from build123d import *

# Parameters (mm, degrees)
F1_DEPTH = 41.275
F2_R     = 5.08
F3_R     = 9.525
F4_R     = 6.35
F5_DEPTH = 55.5635
F6_R     = 6.35
F7_DEPTH = 25.4
F8_W     = 203.2
F8_H     = 76.2
F8_R     = 7.9375
F9_DEPTH = 6.35


with BuildPart() as f1:
    # F0 (on Front) → F1 (new body, symmetric)
    with BuildSketch(Plane.XZ):
        Polygon((21.43125, 21.43125), (21.43125, -21.43125), (-21.43125, -21.43125), (-21.43125, 21.43125), (-27.78125, 21.43125), (-27.78125, -21.43125), (-27.78125, -27.78125), (-21.43125, -27.78125), (21.43125, -27.78125), (27.78125, -27.78125), (27.78125, -21.43125), (27.78125, 21.43125), align=None)
    extrude(amount=F1_DEPTH, both=True)

    # F2
    f2_edges = [f1.edges().sort_by_distance(p)[0] for p in [
        (-21.43125, 0, -21.43125),
        (21.43125, 0, -21.43125),
    ]]
    fillet(f2_edges, radius=F2_R)

    # F3
    f3_edges = [f1.edges().sort_by_distance(p)[0] for p in [
        (-27.78125, 0, -27.78125),
        (27.78125, 0, -27.78125),
    ]]
    fillet(f3_edges, radius=F3_R)

    # F4 (on face) → F5 (cut, through all)
    with BuildSketch(Plane.YZ.offset(27.78125)):
        with Locations((-20.6375, 0)):
            Circle(F4_R)
        with Locations((20.6375, 0)):
            Circle(F4_R)
    extrude(amount=-F5_DEPTH, mode=Mode.SUBTRACT)

    # F6 (on face) → F7 (cut)
    with BuildSketch(Plane(origin=(0, 0, -27.78125), x_dir=(1, 0, 0), z_dir=(0, 0, -1))):
        with Locations((0, 20.6375)):
            Circle(F6_R)
        with Locations((0, -20.6375)):
            Circle(F6_R)
    extrude(amount=-F7_DEPTH, mode=Mode.SUBTRACT)

    # F8 (on face) → F9 (join)
    with BuildSketch(Plane(origin=(0, 41.275, 0), x_dir=(-1, 0, 0), z_dir=(0, 1, 0))):
        with Locations((0, -16.66875)):
            Rectangle(F8_W, F8_H)
        with Locations((-79.375, -16.66875)):
            Circle(F8_R, mode=Mode.SUBTRACT)
        with Locations((79.375, -16.66875)):
            Circle(F8_R, mode=Mode.SUBTRACT)
    extrude(amount=F9_DEPTH)


solid = f1.part
The listing builds one solid part. Answer for the finished solid, in the listing's coordinates (mm). A direction names the side the tool comes from. Coordinates: 2 decimals unless noted, no trailing zeros. Loops run counter-clockwise (first coordinate to the right, second up) from the corner with the lowest first, then second, coordinate; pieces in that order, holes last.
1) A tool of negligible diameter and unlimited length cuts with its end or side. For faces 4 (the face through (-24.917, -0.578, -25.065)), 5 (the face through (27.781, -1, 1)), 6 (the face through (0, -1, -27.781)), 7 (the face through (-27.781, -1, 2)), 8 (the face through (1, 41.275, -33)), from which of +Z, -Z, +X, -X, +Y, -Y can it reach the whole face along a straight path? Write none if from no direction.
2) Find section B-B on x = 0. Write down the section's boundary in (y, z) (1 decimal).
3) Flat-ended cylindrical pins translate along their axes: pin 1 Ø14.5 at (x, y) = (0, -20.64) entering from -Z; pin 2 Ø21.5 at (x, z) = (-5, -3.5) entering from -Y (3 decimals); pin 3 Ø10 at (x, y) = (-1, -15) entering from +Z; pin 4 Ø10 at (y, z) = (20.64, 0) entering from -X. Find the tip coordinate at first contact, or state that the pin passes through.
4) Determine the mould class of faces 1 (the face through (0, 41.275, 0)), 2 (the face through (1, 44, -54.769)), 3 (the face through (87.305, 44.406, -16.32)) for opening direction Z: pulls with the +Z half, pulls with the -Z half, needs draft (parallel to the pull), parting line crosses it, or undercut.
5) Find section A-A on z = 0. Write down the section's boundary in (x, y) (1 decimal), then the cut area to 3 significant figures.
6) Find section C-C on y = 36.5. Write down the section's boundary in (x, z) (3 decimals), then the cut area to 3 significant figures.
7) Find the intervals of material crossed by L1, parallel to Y at x = 0, z = -26 (1 decimal); L2, parallel to X at y = 22, z = 9; L3, parallel to Y at x = 39, z = 1.5 (3 decimals), in increasing order.
8) Find section D-D on x = -74. Write down the section's boundary in (y, z) (3 decimals).
Values:
1. face 4: -Z, -X, -Y
1. face 5: +Z, -Z, +X, -Y
1. face 6: -Z, +X, -X, -Y
1. face 7: +Z, -Z, -X, -Y
1. face 8: -Z, -Y
2. outline: (-41.3, -27.8) - (-27, -27.8) - (-27, -21.4) - (-41.3, -21.4) - close; (-14.3, -27.8) - (14.3, -27.8) - (14.3, -21.4) - (-14.3, -21.4) - close; (27, -27.8) - (41.3, -27.8) - (41.3, -54.8) - (47.6, -54.8) - (47.6, 21.4) - (41.3, 21.4) - (41.3, -21.4) - (27, -21.4) - close
3. pin 1: stops at z = -27.78
3. pin 2: stops at y = 41.275
3. pin 3: stops at z = -21.43
3. pin 4: passes through
4. face 1: needs draft
4. face 2: pulls with the -Z half
4. face 3: undercut
5. outline: (-101.6, 41.3) - (-27.8, 41.3) - (-27.8, 27) - (-21.4, 27) - (-21.4, 41.3) - (21.4, 41.3) - (21.4, 27) - (27.8, 27) - (27.8, 41.3) - (101.6, 41.3) - (101.6, 47.6) - (-101.6, 47.6) - close; (-27.8, -41.3) - (-21.4, -41.3) - (-21.4, -27) - (-27.8, -27) - close; (-27.8, -14.3) - (-21.4, -14.3) - (-21.4, 14.3) - (-27.8, 14.3) - close; (21.4, -41.3) - (27.8, -41.3) - (27.8, -27) - (21.4, -27) - close; (21.4, -14.3) - (27.8, -14.3) - (27.8, 14.3) - (21.4, 14.3) - close
5. area: 2,020 mm2
6. outline: (-27.781, -18.256) arc R9.525 ccw to (-18.256, -27.781) - (18.256, -27.781) arc R9.525 ccw to (27.781, -18.256) - (27.781, 21.431) - (21.431, 21.431) - (21.431, -16.351) arc R5.08 cw to (16.351, -21.431) - (-16.351, -21.431) arc R5.08 cw to (-21.431, -16.351) - (-21.431, 21.431) - (-27.781, 21.431) - close
6. area: 869 mm2
7. L1: y = -41.3 to -27, -14.3 to 14.3, 27 to 47.6
7. L2: x = -27.78 to -21.43, 21.43 to 27.78
7. L3: y = 41.275 to 47.625
8. outline: (41.275, -54.769) - (47.625, -54.769) - (47.625, -22.509) - (41.275, -22.509) - close; (41.275, -10.828) - (47.625, -10.828) - (47.625, 21.431) - (41.275, 21.431) - close
